Geometry: final body of the model. Coordinates: model frame, mm. A direction names the side the tool comes from. Coordinates: 2 decimals unless noted, no trailing zeros. Order: outer loops, then holes, each group sorted by start corner. A loop starts at its lowest first (then second) coordinate and runs counter-clockwise, first axis right, second up. Notation, with made-up numbers: (63, 71) - (97, 71) arc R15 cw to (97, 81) - close; hole circle Ø10 at (23.5, 12.5). An arc over 180 degrees is marked (long way). Use a Markdown table: item, result. Add a question column.
```python
from build123d import *

# Parameters (mm, degrees)
F0_R      = 12
F1_DEPTH  = 8
F2_R      = 1
F3_R      = 8
F4_DEPTH  = 105
F6_R      = 8
F7_DEPTH  = 1
F8_SIZE   = 1
F9_R      = 2
F10_DEPTH = 12.5


with BuildPart() as f1:
    # F0 (on Right) → F1 (new body)
    with BuildSketch(Plane.YZ):
        Circle(F0_R)
    extrude(amount=F1_DEPTH)

    # F2
    f2_edges = [f1.edges().sort_by_distance(p)[0] for p in [
        (0, -12, 0),
    ]]
    fillet(f2_edges, radius=F2_R)

    # F3 (on face) → F4 (join)
    with BuildSketch(Plane.YZ.offset(8)):
        Circle(F3_R)
    extrude(amount=F4_DEPTH)

    # F6 (on face) → F7 (join)
    with BuildSketch(Plane.YZ.offset(113)):
        Circle(F6_R)
    extrude(amount=F7_DEPTH)

    # F8
    f8_edges = [f1.edges().sort_by_distance(p)[0] for p in [
        (114, -8, 0),
    ]]
    chamfer(f8_edges, length=F8_SIZE)

    # F9 (on Front) → F10 (cut, symmetric)
    with BuildSketch(Plane.XZ):
        with Locations((102, 0)):
            Circle(F9_R)
    extrude(amount=F10_DEPTH, both=True, mode=Mode.SUBTRACT)


solid = f1.part
```
1) Pin query (flat end, axial travel): pin 1 (10 mm diameter, centred on x = 98, z = -2.5, fed in from +Y); pin 2 (8 mm diameter, centred on x = 47, z = -8.5, fed in from -Y); pin 3 (5 mm diameter, centred on x = 101.5, y = -8.5, fed in from +Z). Return the tip coordinate at first contact, or that it passes through.
2) Section C-C (x = 34). Return loops of the section in (y, z).
3) Ray query, line 1 along X through (y, z) = (-2.5, 0); line 2 along X through (y, z) = (-3, -10.5); line 3 along Z through (x, y) = (102, -4.5). Return the intervals inside material, ascending.
4) Draft query along X for faces 3 (the face through (103.908, -0.112, 0.601)), 4 (the face through (4.45, -11.99, 0.53)), 5 (the face through (114, 0, 0)). Return one class per face: pulls with the +X half, pulls with the -X half, needs draft (parallel to the pull), parting line crosses it, or undercut.
5) Set-up query: faces 1 (the face through (8, 2, -8)), 2 (the face through (0, 0, 0)). Return all of +Z, -Z, +X, -X, +Y, -Y with unobstructed straight access to the full face (end or side cutting, diameter ignored); none if empty.
6) Section A-A (y = 0). Return loops of the section in (x, z), then the cut area to 3 significant figures.
7) Section B-B (z = 0). Return loops of the section in (x, y).
8) Section D-D (x = 102). Return loops of the section in (y, z).
Values follow:
| question | item | result |
|---|---|---|
| 1 | pin 1 | stops at y = 8 |
| 1 | pin 2 | stops at y = -6.61 |
| 1 | pin 3 | stops at z = 5.29 |
| 2 | outline | circle Ø16 at (0, 0) |
| 3 | line 1 | x = 0 to 100, 104 to 114 |
| 3 | line 2 | x = 0 to 8 |
| 3 | line 3 | z = -6.61 to -2, 2 to 6.61 |
| 4 | face 3 | undercut |
| 4 | face 4 | needs draft |
| 4 | face 5 | pulls with the +X half |
| 5 | face 1 | +X |
| 5 | face 2 | +Z, -Z, -X, +Y, -Y |
| 6 | outline | (0, -11) arc R1 ccw to (1, -12) - (8, -12) - (8, -8) - (113, -8) - (114, -7) - (114, 7) - (113, 8) - (8, 8) - (8, 12) - (1, 12) arc R1 ccw to (0, 11) - close; hole circle Ø4 at (102, 0) |
| 6 | area | 1,870 mm² |
| 7 | outline | (0, -11) arc R1 ccw to (1, -12) - (8, -12) - (8, -8) - (100, -8) - (100, 8) - (8, 8) - (8, 12) - (1, 12) arc R1 ccw to (0, 11) - close; (104, -8) - (113, -8) - (114, -7) - (114, 7) - (113, 8) - (104, 8) - close |
| 8 | outline | (-7.75, -2) arc R8 ccw to (7.75, -2) - close; (-7.75, 2) - (7.75, 2) arc R8 ccw to start |
